For this review, take the finished solid that the model builds, in its own axes (mm). Face numbers are marked on the shaded views. A direction names the side the tool comes from. Round coordinates to 2 decimals unless told otherwise and drop trailing zeros. Write each loop counter-clockwise with the first axis right and the second up, starting at its lowest first coordinate (ties: lowest second). Pieces come first, ordered by that corner, then holes. Notation, with made-up numbers: (70.5, -34.5) -> (129.5, -34.5) arc R16 ccw to (129.5, -7.5) -> close; hole circle Ø3 at (73.25, -38). An arc over 180 degrees is marked (long way). Write each question's results on one line, items separated by ' | '. Start each with the question number.
Item 1: Add section B-B (z = 4.5). State the section outline as (x, y) points, plus the area to 3 significant figures.
Item 2: Add section C-C (x = 64.5). State the section outline as (y, z) points, plus the area to 3 significant figures.
Item 3: To check wall thickness, follow line 1 along Z through (x, y) = (64.5, 4); line 2 along X through (y, z) = (2.75, 4.5); line 3 along Z through (x, y) = (64, 3). State the ranges of each line that lie inside material, in increasing order.
Item 4: Tool access review of the marked faces 1, 2 and 3: name each direction out of +Z, -Z, +X, -X, +Y, -Y from which nothing blocks a thin tool from reaching the whole face with its end or side.
Item 5: Clearance check with flat-ended pins moving along their axes: pin 1 (3 mm diameter, centred on x = 22.5, y = 5, fed in from +Z); pin 2 (3.5 mm diameter, centred on y = 2.5, z = -9.5, fed in from -X); pin 3 (3 mm diameter, centred on x = 43.5, y = 6, fed in from -Z). State where each tip first meets the part, or that it passes through.
Item 6: Add section A-A (y = 3.5). State the section outline as (x, z) points, plus the area to 3 significant figures.
Item 7: Add section D-D (z = -1.5). State the section outline as (x, y) points.
from build123d import *

# Parameters (mm, degrees)
SKETCH1_R           = 1.5
SKETCH1_W           = 60
SKETCH1_H           = 7
BOSS_EXTRUDE1_DEPTH = 7
SKETCH2_R           = 2
CUT_EXTRUDE1_DEPTH  = 7


with BuildPart() as part:
    # Sketch1 → Boss-Extrude1 (new body)
    with BuildSketch(Plane(origin=(0, 0, 0), x_dir=(1, 0, 0), z_dir=(0, 1, 0))):
        Polygon((60, 7), (60, 0), (60, -9), (69, -9), (69, 16), (60, 16), align=None)
        with Locations((64.5, -4.5)):
            Circle(SKETCH1_R, mode=Mode.SUBTRACT)
        with Locations((64.5, 11.5)):
            Circle(SKETCH1_R, mode=Mode.SUBTRACT)
        with Locations((30, 3.5)):
            Rectangle(SKETCH1_W, SKETCH1_H)
    extrude(amount=BOSS_EXTRUDE1_DEPTH)

    # Sketch2 → Cut-Extrude1 (cut)
    with BuildSketch(Plane(origin=(0, 0, -7), x_dir=(-1, 0, 0), z_dir=(0, 0, -1))):
        with Locations((-4.944972507, 3.5)):
            Circle(SKETCH2_R)
    extrude(amount=-CUT_EXTRUDE1_DEPTH, mode=Mode.SUBTRACT)


solid = part.part
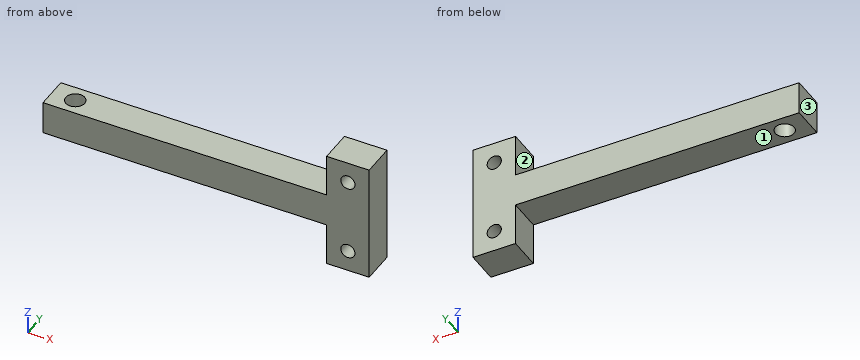
Responses:
1) outline: (60, 0) -> (63, 0) -> (63, 7) -> (60, 7) -> close; (66, 0) -> (69, 0) -> (69, 7) -> (66, 7) -> close | area: 42.0 mm^2
2) outline: (0, -16) -> (7, -16) -> (7, -13) -> (0, -13) -> close; (0, -10) -> (7, -10) -> (7, 3) -> (0, 3) -> close; (0, 6) -> (7, 6) -> (7, 9) -> (0, 9) -> close | area: 133 mm^2
3) line 1: z = -16 to -13, -10 to 3, 6 to 9 | line 2: x = 60 to 63, 66 to 69 | line 3: z = -16 to -12.91, -10.09 to 3.09, 5.91 to 9
4) face 1: -Z, -X, +Y, -Y | face 2: +Z, -X, +Y, -Y | face 3: +Z, -Z, -X, +Y, -Y
5) pin 1: stops at z = 0 | pin 2: stops at x = 60 | pin 3: stops at z = -7
6) outline: (0, -7) -> (2.94, -7) -> (2.94, 0) -> (0, 0) -> close; (6.94, -7) -> (60, -7) -> (60, -16) -> (69, -16) -> (69, 9) -> (60, 9) -> (60, 0) -> (6.94, 0) -> close; hole circle Ø3 at (64.5, -11.5); hole circle Ø3 at (64.5, 4.5) | area: 603 mm^2
7) outline: (0, 0) -> (69, 0) -> (69, 7) -> (0, 7) -> close; hole circle Ø4 at (4.94, 3.5)
